The model under review builds one solid part; all positions refer to its coordinate system, in mm. Face numbers are marked on the shaded views. A direction names the side the tool comes from. Coordinates: 2 decimals unless noted, no trailing zeros. Write each loop counter-clockwise with the first axis right and the second up, starting at its lowest first coordinate (ties: lowest second). Pieces come first, ordered by that corner, then holes. Notation, with made-up numbers: (75, 5) -> (110, 5) arc R19 cw to (110, 19) -> close; hole circle Ø2 at (-15, 69.25). An arc over 180 degrees is marked (long way). Write each question's results on one line, items separated by ' | '.
```python
from build123d import *

# Parameters (mm, degrees)
POCKET_DEPTH       = 5
POLARPATTERN_COUNT = 4


with BuildPart() as part:
    # Sketch → Revolution (revolve)
    with BuildSketch(Plane.XY):
        Polygon((-2.05, 5), (-2.05, -5), (-16, -5), (-16, -4), (-15, -4), (-15, 4), (-16, 4), (-16, 5), (-13.5, 5), (-13.5, -1), (-11, -3.5), (-6.05, -3.5), (-3.55, -1), (-3.55, 5), align=None)
    revolve(axis=Axis((0, 0, 0), (0, 1, 0)))

    # Sketch001 → Pocket (cut)
    with BuildSketch(Plane.XZ.offset(5)):
        with BuildLine():
            ThreePointArc((-1.5, 3.708099), (-2.828427, 2.828427), (-3.708099, 1.5))
            Line((-12.913172, 1.5), (-3.708099, 1.5))
            ThreePointArc((-1.5, 12.913172), (-9.192388, 9.192388), (-12.913172, 1.5))
            Line((-1.5, 12.913172), (-1.5, 3.708099))
        make_face()
    pocket = extrude(amount=-POCKET_DEPTH, mode=Mode.SUBTRACT)

    # PolarPattern: Pocket ×4 about axis
    polarpattern_axis = Axis((0, -5, 0), (0, -1, 0))
    for i in range(1, POLARPATTERN_COUNT):
        add(pocket.rotate(polarpattern_axis, i * 360 / POLARPATTERN_COUNT), mode=Mode.SUBTRACT)


solid = part.part
```
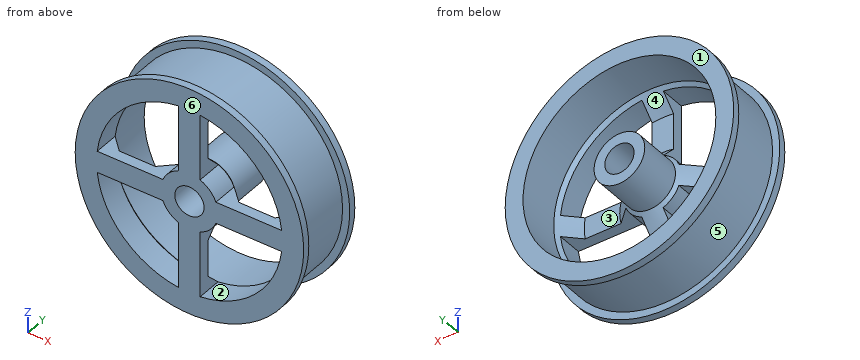
Q1. Add section B-B (x = 0). Write out the cut boundary in (y, z), plus the area to 3 significant figures.
Solution:
outline: (-5, -16) -> (-4, -16) -> (-4, -15) -> (4, -15) -> (4, -16) -> (5, -16) -> (5, -13.5) -> (-1, -13.5) -> (-3.5, -11) -> (-3.5, -6.05) -> (-1, -3.55) -> (5, -3.55) -> (5, -2.05) -> (-5, -2.05) -> close; (-5, 2.05) -> (5, 2.05) -> (5, 3.55) -> (-1, 3.55) -> (-3.5, 6.05) -> (-3.5, 11) -> (-1, 13.5) -> (5, 13.5) -> (5, 16) -> (4, 16) -> (4, 15) -> (-4, 15) -> (-4, 16) -> (-5, 16) -> close | area: 106 mm²
Q2. For line 1 (Z direction, x = 0, y = 2.1); line 2 (Y direction, x = 11, z = -10.5); line 3 (Z direction, x = 11.5, y = -3.75), list the stretches that pass through material, from the lowest coordinate up. Write a range as from..to.
Solution:
line 1: -15..-13.5, -3.55..-2.05, 2.05..3.55, 13.5..15 | line 2: -5..-4, 4..5 | line 3: -9.63..-6.06, -1.5..1.5, 6.06..9.63
Q3. Add section D-D (z = -8.5). Count the separate pieces of the cut face and the enclosed holes in it, plus the area to 3 significant figures.
Solution:
separate pieces: 3 | enclosed holes: 0 | area: 51.6 mm²
Q4. Clearance check with flat-ended pins moving along their axes: P1, Ø3, axis at x = -8.5, y = 0, coming from the -Z side; P2, Ø1.5, axis at x = 0, z = 8, coming from the +Y side; P3, Ø4, axis at x = 6.5, y = -3.5, coming from the +Z side; P4, Ø1, axis at x = 9, z = 3.5, coming from the -Y side. State where each tip first meets the part, or that it passes through.
Solution:
P1: z = -13.27 | P2: y = -3.5 | P3: z = 15.34 | P4: through
Q5. Add section A-A (z = 0). Write out the cut boundary in (x, y).
Solution:
outline: (-16, -5) -> (-2.05, -5) -> (-2.05, 5) -> (-3.55, 5) -> (-3.55, -1) -> (-6.05, -3.5) -> (-11, -3.5) -> (-13.5, -1) -> (-13.5, 5) -> (-16, 5) -> (-16, 4) -> (-15, 4) -> (-15, -4) -> (-16, -4) -> close; (2.05, -5) -> (16, -5) -> (16, -4) -> (15, -4) -> (15, 4) -> (16, 4) -> (16, 5) -> (13.5, 5) -> (13.5, -1) -> (11, -3.5) -> (6.05, -3.5) -> (3.55, -1) -> (3.55, 5) -> (2.05, 5) -> close
Q6. Draft analysis for pull direction Z (two halves, no side actions). For the marked faces 4, 5 and 6, state which applies: pulls with the +Z half, pulls with the -Z half, needs draft (parallel to the pull), parting line crosses it, or undercut.
Solution:
face 4: undercut | face 5: parting line crosses it | face 6: needs draft
Q7. Machinability: for the marked faces 1, 2 and 3, which of the approach directions +Z, -Z, +X, -X, +Y, -Y give a long, thin tool a straight path to every point of the face, cutting with its end or side? Answer none if there is none.
Solution:
face 1: +Z, -Z, +X, -X, +Y | face 2: +Y, -Y | face 3: +Y
Q8. Add section C-C (y = 2.75). Write out the cut boundary in (x, z), plus the area to 3 significant figures.
Solution:
outline: circle Ø30 at (0, 0); circle Ø7.1 at (0, 0); hole circle Ø27 at (0, 0); hole circle Ø4.1 at (0, 0) | area: 161 mm²
